Here's how the part is built. I have some questions about the finished solid (model axes, mm). A direction names the side the tool comes from. Coordinates: 2 decimals unless noted, no trailing zeros. Loops run counter-clockwise (first coordinate to the right, second up) from the corner with the lowest first, then second, coordinate; pieces in that order, holes last. Notation, with made-up numbers: (78, 49.5) -> (96, 49.5) arc R3 ccw to (96, 53.5) -> close; hole circle Ø4 at (10.5, 79.25). An arc over 180 degrees is marked (long way). Answer as a JSON object with one key per item and string values. Group by question number.
1) I want a section at A-A (y = 193). Write out the boundary of the cut face in (x, z), then the cut area to 3 significant figures.
2) I want a section at D-D (y = 54). Write out the boundary of the cut face in (x, z), then the cut area to 3 significant figures.
3) I'm going to push flat-ended pins straight in: pin 1 (0.9 mm diameter, centred on x = 248, y = 199, fed in from -Z); pin 2 (3 mm diameter, centred on x = -165.5, y = -36, fed in from +Z); pin 3 (0.9 mm diameter, centred on x = 249, z = 332, fed in from -Y); pin 4 (8 mm diameter, centred on x = -26.5, z = 499, fed in from -Y). Where does each tip first touch, or does it pass through?
4) I want a section at B-B (x = 135). Write out the boundary of the cut face in (y, z).
5) I want a section at C-C (z = 448.5). Write out the boundary of the cut face in (x, y).
6) Which directions (+Z, -Z, +X, -X, +Y, -Y) give clear straight access to the entire face, cutting with the end or side of a thin tool? Please do faces 5 (the flat face through (-3, 0, 8)), 6 (the flat face through (-3, 250, 248)).
7) I need wall thicknesses on probe 1 along Z at (x, y) = (19, 150.5); probe 2 along Z at (x, y) = (193.5, 118); probe 3 along Y at (x, z) = (-95, 62.5). Which ranges of each line are inside material? Lowest first, please. Write a range as [from, to].
8) If we mould it in two halves opening along Z, with no side actions, what happens to faces 1 (the flat face through (-3, 192, 493)), 2 (the flat face through (-3, 198, 503)), 3 (the flat face through (-3, 240, 254)), 4 (the flat face through (-3, 4, 0))? For each: +Z half, -Z half, draft (parallel to the pull), parting line (faces both ways), or undercut.
```python
from build123d import *

# Parameters (mm, degrees)
F0_W      = 500
F0_H      = 500
F1_DEPTH  = 3
F2_W      = 494
F2_H      = 492
F3_DEPTH  = 5
F4_W      = 500
F4_H      = 5
F5_DEPTH  = 500
F6_W      = 494
F6_H      = 490
F7_DEPTH  = 5
F8_W      = 500
F8_H      = 5
F9_DEPTH  = 100
F10_W     = 494
F10_H     = 95
F12_DEPTH = 5


with BuildPart() as f1:
    # F0 (on Top) → F1 (new body)
    with BuildSketch(Plane.XY):
        Rectangle(F0_W, F0_H)
    extrude(amount=F1_DEPTH)

    # F2 (on face) → F3 (join)
    with BuildSketch(Plane.XY.offset(3)):
        with Locations((0, -1)):
            Rectangle(F2_W, F2_H)
    extrude(amount=F3_DEPTH)

    # F4 (on face) → F5 (join)
    with BuildSketch(Plane.XY.offset(3)):
        with Locations((0, 247.5)):
            Rectangle(F4_W, F4_H)
    extrude(amount=F5_DEPTH)

    # F6 (on face) → F7 (join)
    with BuildSketch(Plane.XZ.offset(-245)):
        with Locations((0, 253)):
            Rectangle(F6_W, F6_H)
    extrude(amount=F7_DEPTH)

    # F8 (on face) → F9 (join)
    with BuildSketch(Plane.XZ.offset(-245)):
        with Locations((0, 500.5)):
            Rectangle(F8_W, F8_H)
    extrude(amount=F9_DEPTH)

    # F10 (on face) → F12 (join)
    with BuildSketch(Plane(origin=(0, 0, 498), x_dir=(1, 0, 0), z_dir=(0, 0, -1))):
        with Locations((0, -192.5)):
            Rectangle(F10_W, F10_H)
    extrude(amount=F12_DEPTH)


solid = f1.part
```
Determined:
{
 "1": {"outline": "(-250, 0) -> (250, 0) -> (250, 3) -> (247, 3) -> (247, 8) -> (-247, 8) -> (-247, 3) -> (-250, 3) -> close; (-250, 498) -> (-247, 498) -> (-247, 493) -> (247, 493) -> (247, 498) -> (250, 498) -> (250, 503) -> (-250, 503) -> close", "area": "8,940 mm^2"},
 "2": {"outline": "(-250, 0) -> (250, 0) -> (250, 3) -> (247, 3) -> (247, 8) -> (-247, 8) -> (-247, 3) -> (-250, 3) -> close", "area": "3,970 mm^2"},
 "3": {"pin 1": "z = 0", "pin 2": "z = 8", "pin 3": "y = 245", "pin 4": "y = 145"},
 "4": {"outline": "(-250, 0) -> (250, 0) -> (250, 503) -> (145, 503) -> (145, 493) -> (240, 493) -> (240, 8) -> (-247, 8) -> (-247, 3) -> (-250, 3) -> close"},
 "5": {"outline": "(-250, 245) -> (-247, 245) -> (-247, 240) -> (247, 240) -> (247, 245) -> (250, 245) -> (250, 250) -> (-250, 250) -> close"},
 "6": {"face 5": "+X, -X, -Y", "face 6": "+Z, -Z, +X, -X, +Y"},
 "7": {"probe 1": "[0, 8], [493, 503]", "probe 2": "[0, 8]", "probe 3": "[240, 250]"},
 "8": {"face 1": "undercut", "face 2": "+Z half", "face 3": "undercut", "face 4": "-Z half"}
}
